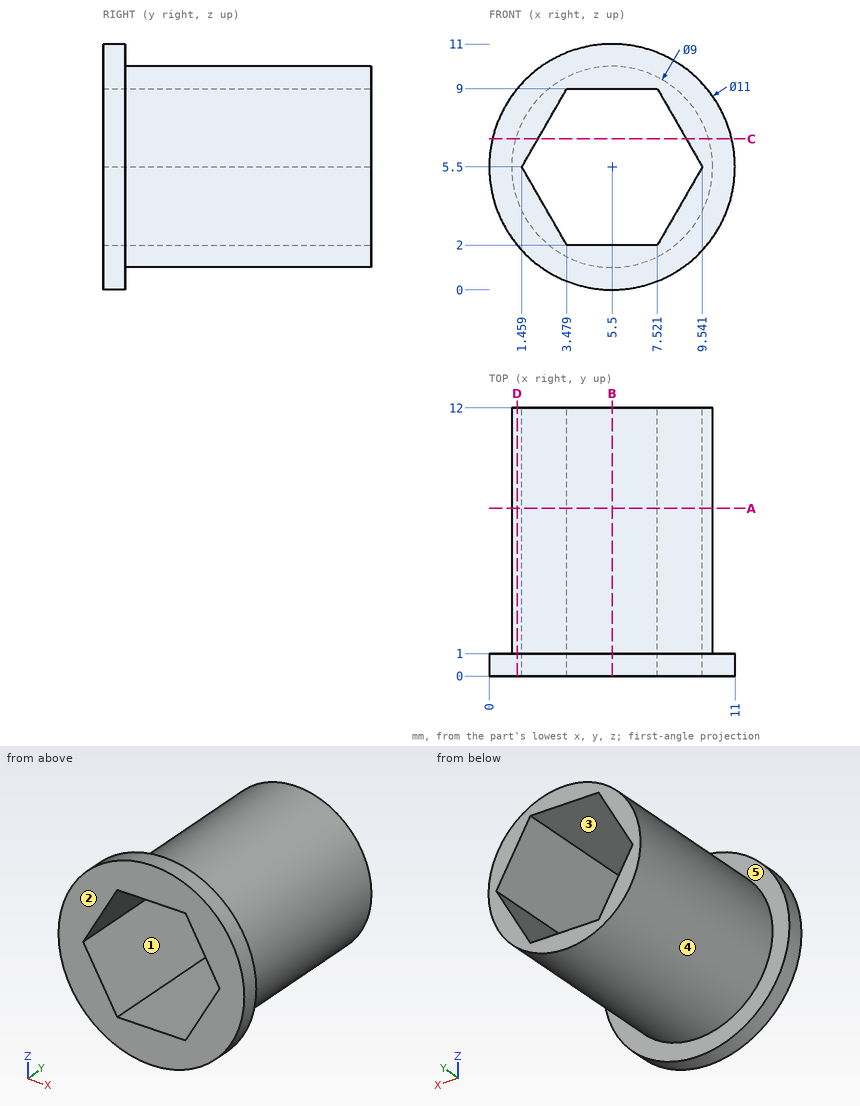
Design review of the part shown in the three views and the two pictorial views. Dimensions are in mm from the part's minimum x, y and z. A direction names the side the tool comes from. Round coordinates to 2 decimals unless told otherwise and drop trailing zeros. Loops run counter-clockwise (first coordinate to the right, second up) from the corner with the lowest first, then second, coordinate; pieces in that order, holes last.
Q1. Add section B-B on x = 5.5. Write out the cut boundary in (y, z).
Result sheet:
outline: (0, 0) - (1, 0) - (1, 1) - (12, 1) - (12, 2) - (0, 2) - close; (0, 9) - (12, 9) - (12, 10) - (1, 10) - (1, 11) - (0, 11) - close
Q2. Add section A-A on y = 7.5. Write out the cut boundary in (x, z).
Result sheet:
outline: circle Ø9 at (5.5, 5.5); hole (1.46, 5.5) - (3.48, 2) - (7.52, 2) - (9.54, 5.5) - (7.52, 9) - (3.48, 9) - close
Q3. Machinability: for the marked faces 1 and 2, which of the approach directions +Z, -Z, +X, -X, +Y, -Y give a long, thin tool a straight path to every point of the face, cutting with its end or side? Answer none if there is none.
Result sheet:
face 1: +Y, -Y
face 2: +Z, -Z, +X, -X, -Y
Q4. To check wall thickness, follow line 1 along Z through (x, y) = (5.5, 10); line 2 along Z through (x, y) = (6.25, 5); line 3 along Y through (x, z) = (1.75, 9). State the ranges of each line that lie inside material, in increasing order.
Result sheet:
line 1: z = 1 to 2, 9 to 10
line 2: z = 1.06 to 2, 9 to 9.94
line 3: y = 0 to 1
Q5. Mouldability with a two-part tool opening along Z and no side actions: class the marked faces 3, 4 and 5 as +Z half, -Z half, draft (parallel to the pull), parting line (faces both ways), or undercut.
Result sheet:
face 3: undercut
face 4: parting line
face 5: draft
Q6. Add section D-D on x = 1.25. Write out the cut boundary in (y, z).
Result sheet:
outline: (0, 2.01) - (1, 2.01) - (1, 4.02) - (12, 4.02) - (12, 6.98) - (1, 6.98) - (1, 8.99) - (0, 8.99) - close
Q7. Add section C-C on z = 6.75. Write out the cut boundary in (x, y).
Result sheet:
outline: (0.14, 0) - (2.18, 0) - (2.18, 12) - (1.18, 12) - (1.18, 1) - (0.14, 1) - close; (8.82, 0) - (10.86, 0) - (10.86, 1) - (9.82, 1) - (9.82, 12) - (8.82, 12) - close
Q8. Insertion check: pin 1 Ø1.5 at (y, z) = (2.5, 8.5) entering from +X; pin 2 Ø3 at (x, y) = (6, 3.5) entering from -Z; pin 3 Ø1.5 at (x, y) = (1.5, 1.5) entering from -Z. Each pin has a flat end and moves straight along its axis. Give the tip position at first contact, or say it passes through.
Result sheet:
pin 1: stops at x = 9.4
pin 2: stops at z = 1
pin 3: stops at z = 1.21
